Can you work these out from the model? Positions are in its coordinate system, mm. Round coordinates to 2 decimals unless told otherwise and drop trailing zeros. Write each loop counter-clockwise with the first axis right and the second up, starting at its lowest first coordinate (ties: lowest second). Pieces come first, ordered by that corner, then holes.
Q1. If we section it at C-C (x = 38.5): Please give me the cut outline in (y, z) (3 decimals), plus the area to 3 significant figures.
Q2. Please list where these lines run through material, in increasing order: line 1 along Z through (x, y) = (68.58, 1.4); line 2 along Z through (x, y) = (47, 0.6); line 3 along Z through (x, y) = (35.5, 1.2).
Q3. If we section it at D-D (y = 2.35): Please give me the cut outline in (x, z).
Q4. If we section it at A-A (z = -27): Please give me the cut outline in (x, y) (3 decimals).
Q5. If we section it at B-B (x = 68.58): Please give me the cut outline in (y, z) (3 decimals).
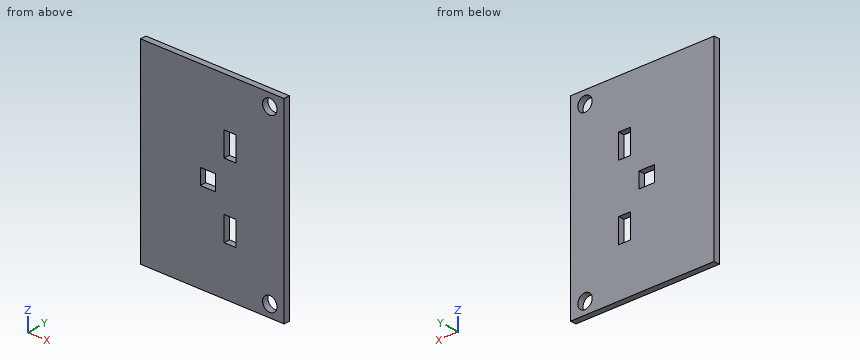
from build123d import *

# Parameters (mm, degrees)
SKETCH1_W           = 76.2
SKETCH1_H           = 101.6
BOSS_EXTRUDE1_DEPTH = 3.175
SKETCH2_R           = 3.81
SKETCH2_W           = 6.35
SKETCH2_H           = 12.7
SKETCH2_W_2         = 8.128
SKETCH2_H_2         = 8.128
CUT_EXTRUDE1_DEPTH  = 4.175


with BuildPart() as part:
    # Sketch1 → Boss-Extrude1 (new body)
    with BuildSketch(Plane(origin=(0, 0, 0), x_dir=(1, 0, 0), z_dir=(0, 1, 0))):
        with Locations((38.1, 50.8)):
            Rectangle(SKETCH1_W, SKETCH1_H)
    extrude(amount=BOSS_EXTRUDE1_DEPTH)

    # Sketch2 → Cut-Extrude1 (cut, through all)
    with BuildSketch(Plane(origin=(0, 3.175, 0), x_dir=(1, 0, 0), z_dir=(0, 1, 0))):
        with Locations((68.58, 95.25)):
            Circle(SKETCH2_R)
        with Locations((68.58, 6.35)):
            Circle(SKETCH2_R)
        with Locations((47.498, 69.85)):
            Rectangle(SKETCH2_W, SKETCH2_H)
        with Locations((47.498, 31.75)):
            Rectangle(SKETCH2_W, SKETCH2_H)
        with Locations((35.814, 50.8)):
            Rectangle(SKETCH2_W_2, SKETCH2_H_2)
    extrude(amount=-CUT_EXTRUDE1_DEPTH, mode=Mode.SUBTRACT)


solid = part.part
A:
1. outline: (0, -101.6) - (3.175, -101.6) - (3.175, -54.864) - (0, -54.864) - close; (0, -46.736) - (3.175, -46.736) - (3.175, 0) - (0, 0) - close
1. area: 297 mm2
2. line 1: z = -101.6 to -99.06, -91.44 to -10.16, -2.54 to 0
2. line 2: z = -101.6 to -76.2, -63.5 to -38.1, -25.4 to 0
2. line 3: z = -101.6 to -54.86, -46.74 to 0
3. outline: (0, -101.6) - (76.2, -101.6) - (76.2, 0) - (0, 0) - close; hole (31.75, -54.86) - (39.88, -54.86) - (39.88, -46.74) - (31.75, -46.74) - close; hole (44.32, -76.2) - (50.67, -76.2) - (50.67, -63.5) - (44.32, -63.5) - close; hole (44.32, -38.1) - (50.67, -38.1) - (50.67, -25.4) - (44.32, -25.4) - close; hole circle Ø7.62 at (68.58, -95.25); hole circle Ø7.62 at (68.58, -6.35)
4. outline: (0, 0) - (44.323, 0) - (44.323, 3.175) - (0, 3.175) - close; (50.673, 0) - (76.2, 0) - (76.2, 3.175) - (50.673, 3.175) - close
5. outline: (0, -101.6) - (3.175, -101.6) - (3.175, -99.06) - (0, -99.06) - close; (0, -91.44) - (3.175, -91.44) - (3.175, -10.16) - (0, -10.16) - close; (0, -2.54) - (3.175, -2.54) - (3.175, 0) - (0, 0) - close
